Geometry check sheet. Reference: drawing and pictorial views, mm from the part's lowest x, y, z. A direction names the side the tool comes from. Round coordinates to 2 decimals unless told otherwise and drop trailing zeros. Order: outer loops, then holes, each group sorted by start corner. A loop starts at its lowest first (then second) coordinate and runs counter-clockwise, first axis right, second up.
(1) Set-up check for the marked faces 1 and 2: record each of +Z, -Z, +X, -X, +Y, -Y from which the full face is reachable in a straight line by a thin tool's end or side.
(2) Sectioned sample at C-C (z = 57). Record the boundary of the cut face in (x, y) (3 decimals).
(3) Sectioned sample at D-D (x = 54). Record the boundary of the cut face in (y, z) (3 decimals), plus the area to 3 significant figures.
(4) Sectioned sample at A-A (y = 76.2). Record the boundary of the cut face in (x, z) (1 decimal), plus the area to 3 significant figures.
(5) Go/stop test with flat-tipped pins: pin 1 (7.5 mm diameter, centred on x = 25.4, y = 152.4, fed in from -Z); pin 2 (5 mm diameter, centred on x = 16, y = 140, fed in from +Z) (3 decimals); pin 3 (1 mm diameter, centred on y = 139.5, z = 9, fed in from -X) (3 decimals); pin 4 (4 mm diameter, centred on x = 25.4, y = 177.8, fed in from -Z). Record where each tip stops, or that it passes through.
(6) Sectioned sample at B-B (y = 114.5). Record the boundary of the cut face in (x, z) (1 decimal), plus the area to 3 significant figures.
(7) Material ranges on line 1 along Z through (x, y) = (18, 40.5) (3 decimals); line 2 along X through (y, z) = (83, 59.5) (3 decimals); line 3 along X through (y, z) = (127, 1) (1 decimal), recorded low to high.
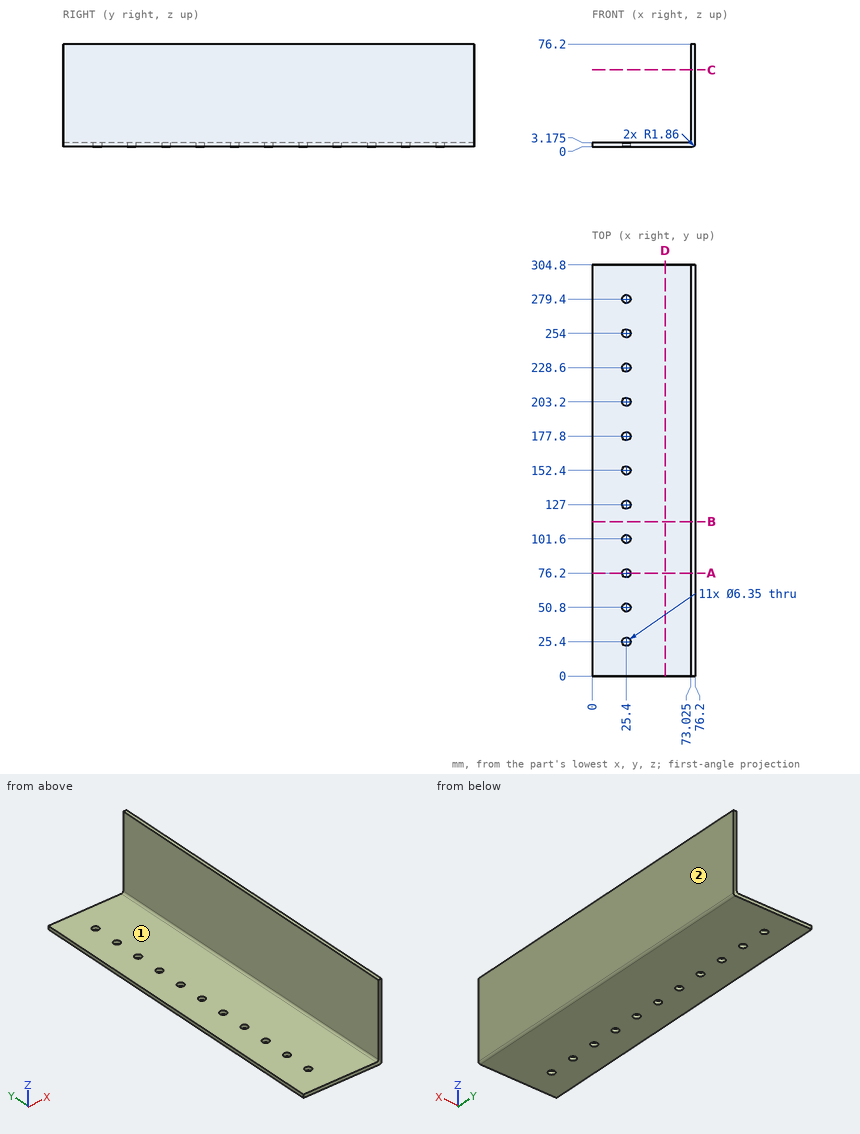
Answer below:
1. face 1: +Z, -X, +Y, -Y
1. face 2: +Z, -Z, +X, +Y, -Y
2. outline: (73.025, 0) - (76.2, 0) - (76.2, 304.8) - (73.025, 304.8) - close
3. outline: (0, 0) - (304.8, 0) - (304.8, 3.175) - (0, 3.175) - close
3. area: 968 mm2
4. outline: (0, 0) - (22.2, 0) - (22.2, 3.2) - (0, 3.2) - close; (28.6, 0) - (74.3, 0) arc R1.9 ccw to (76.2, 1.9) - (76.2, 76.2) - (73, 76.2) - (73, 5) arc R1.9 cw to (71.2, 3.2) - (28.6, 3.2) - close
4. area: 454 mm2
5. pin 1: stops at z = 0
5. pin 2: stops at z = 3.175
5. pin 3: stops at x = 73.025
5. pin 4: passes through
6. outline: (0, 0) - (74.3, 0) arc R1.9 ccw to (76.2, 1.9) - (76.2, 76.2) - (73, 76.2) - (73, 5) arc R1.9 cw to (71.2, 3.2) - (0, 3.2) - close
6. area: 474 mm2
7. line 1: z = 0 to 3.175
7. line 2: x = 73.025 to 76.2
7. line 3: x = 0 to 22.2, 28.6 to 76
